Answer from the drawing. Dimensions are ordinates in mm from the lowest x, y and z of the part. Round coordinates to 2 decimals unless told otherwise and drop trailing zeros. Write each loop counter-clockwise with the first axis right and the second up, starting at its lowest first coordinate (ties: lowest second). Pieces come first, ordered by that corner, then holes. Notation, with made-up numbers: (78, -27) - (112, -27) arc R18 cw to (112, 3) - close; hole circle Ø3 at (31.5, 84). An arc over 180 degrees is marked (long way). Answer as a JSON object with one key per item and string values.
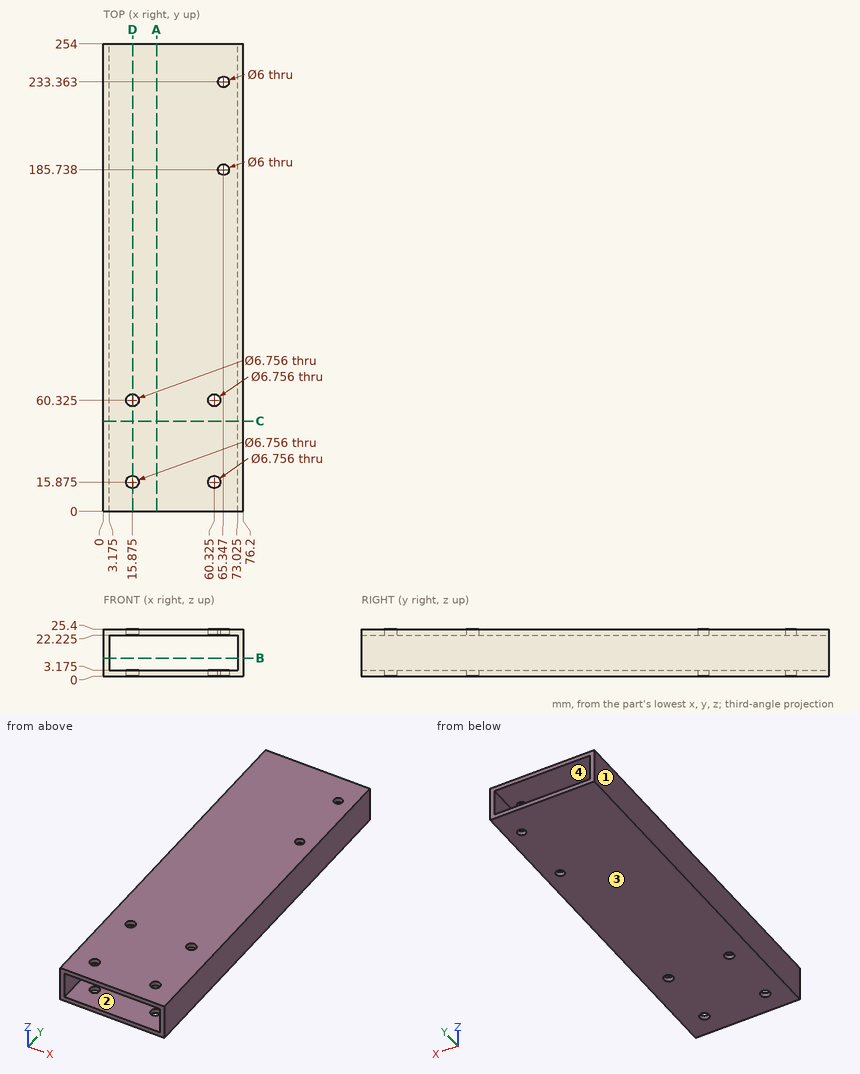
Item 1: A cutting plane is placed at A-A (x = 29). Write down the section's boundary in (y, z) (1 decimal).
Results found:
{"outline": "(0, 0) - (254, 0) - (254, 3.2) - (0, 3.2) - close; (0, 22.2) - (254, 22.2) - (254, 25.4) - (0, 25.4) - close"}
Item 2: A cutting plane is placed at B-B (z = 9.75). Write down the section's boundary in (x, y) (1 decimal), and give its area (3 significant figures).
Results found:
{"outline": "(0, 0) - (3.2, 0) - (3.2, 254) - (0, 254) - close; (73, 0) - (76.2, 0) - (76.2, 254) - (73, 254) - close", "area": "1,610 mm²"}
Item 3: A cutting plane is placed at C-C (y = 49). Write down the section's boundary in (x, z) (1 decimal).
Results found:
{"outline": "(0, 0) - (76.2, 0) - (76.2, 25.4) - (0, 25.4) - close; hole (3.2, 3.2) - (73, 3.2) - (73, 22.2) - (3.2, 22.2) - close"}
Item 4: Consider line 1 along X through (y, z) = (227, 7.25) (1 decimal); line 2 along Z through (x, y) = (48.5, 141) (1 decimal); line 3 along Y through (x, z) = (15, 2). Determine where each line is inside the solid, lowest interval first.
Results found:
{"line 1": "0 to 3.2, 73 to 76.2", "line 2": "0 to 3.2, 22.2 to 25.4", "line 3": "0 to 12.61, 19.14 to 57.06, 63.59 to 254"}
Item 5: A cutting plane is placed at D-D (x = 16). Give the number of separate pieces and of enclosed holes in the cut face, and give its area (3 significant figures).
Results found:
{"separate pieces": "6", "enclosed holes": "0", "area": "1,530 mm²"}
Item 6: This flat-tipped pin is pushed along its axis until it touches: P1, Ø5.5, axis at x = 65.35, y = 185.74, coming from the +Z side. Where does it stop, or does it pass through?
Results found:
{"P1": "through"}
Item 7: Determine the mould class of the marked faces 1, 2, 3 and 4 for opening direction Z: pulls with the +Z half, pulls with the -Z half, needs draft (parallel to the pull), parting line crosses it, or undercut.
Results found:
{"face 1": "needs draft", "face 2": "undercut", "face 3": "pulls with the -Z half", "face 4": "undercut"}
